Source: CAD feature listing. Evaluate the final solid. Frame: model axes, mm. A direction names the side the tool comes from. Coordinates: 2 decimals unless noted, no trailing zeros. Loops run counter-clockwise (first coordinate to the right, second up) from the corner with the lowest first, then second, coordinate; pieces in that order, holes last.
from build123d import *

# Parameters (mm, degrees)
BOSS_EXTRUDE1_DEPTH = 3.175
SKETCH2_R           = 2.5527
CUT_EXTRUDE1_DEPTH  = 77.793005053
SKETCH3_R           = 2.5527
CUT_EXTRUDE2_DEPTH  = 77.793005053


with BuildPart() as part:
    # Sketch1 → Boss-Extrude1 (new body)
    with BuildSketch(Plane(origin=(0, 0, 0), x_dir=(1, 0, 0), z_dir=(0, 1, 0))):
        Polygon((0, 0), (0, 44.45), (-13.97, 44.45), (-13.97, 67.31), (36.83, 67.31), (36.83, 44.45), (22.86, 44.45), (22.86, 0), align=None)
    extrude(amount=BOSS_EXTRUDE1_DEPTH)

    # Sketch2 → Cut-Extrude1 (cut, through all)
    with BuildSketch(Plane(origin=(0, 3.175, 0), x_dir=(1, 0, 0), z_dir=(0, 1, 0))):
        with Locations(Location((-7.62, 57.15, 0), (0, 0, 270))):
            Circle(SKETCH2_R)
        with Locations(Location((5.08, 57.15, 0), (0, 0, 270))):
            Circle(SKETCH2_R)
        with Locations(Location((17.78, 57.15, 0), (0, 0, 270))):
            Circle(SKETCH2_R)
        with Locations(Location((30.48, 57.15, 0), (0, 0, 270))):
            Circle(SKETCH2_R)
    extrude(amount=-CUT_EXTRUDE1_DEPTH, mode=Mode.SUBTRACT)

    # Sketch3 → Cut-Extrude2 (cut, through all)
    with BuildSketch(Plane(origin=(0, 3.175, 0), x_dir=(1, 0, 0), z_dir=(0, 1, 0))):
        with Locations(Location((11.43, 31.75, 0), (0, 0, 270))):
            Circle(SKETCH3_R)
        with Locations(Location((11.43, 19.05, 0), (0, 0, 270))):
            Circle(SKETCH3_R)
        with Locations(Location((11.43, 6.35, 0), (0, 0, 270))):
            Circle(SKETCH3_R)
    extrude(amount=-CUT_EXTRUDE2_DEPTH, mode=Mode.SUBTRACT)


solid = part.part
Q1. Section A-A, the plane x = 11.43. Return the cut outline in (y, z) (3 decimals).
Q2. Contact query for flat-ended pins moving along their axis: pin 1 Ø8 at (x, z) = (11.43, -19.05) entering from +Y (3 decimals); pin 2 Ø1.6 at (x, y) = (-7.5, 2.5) entering from +Z; pin 3 Ø1.6 at (y, z) = (2, -18) entering from -X. Output: stop coordinate, or through.
Q3. Section D-D, the plane x = 17.78. Return the cut outline in (y, z) (3 decimals), plus the area to 4 significant figures.
Q4. Draft query along X for faces 4 (the cylindrical face through (10.452, 1.61, -29.392)), 5 (the flat face through (0, 2, -22)), 6 (the flat face through (12, 3.175, -42)). Return one class per face: +X half, -X half, draft (parallel to the pull), parting line (faces both ways), or undercut.
Q5. Access query for faces 1 (the flat face through (12, 2, 0)), 2 (the flat face through (-7, 2, -44.45)), 3 (the flat face through (22.86, 2, -23)). Directions: +Z, -Z, +X, -X, +Y, -Y. A direction counts if a zero-diameter tool reaches every point of the face in a straight line with its end or side. Return the directions, or none.
Q6. Line query: line 1 along X through (y, z) = (1.6, -57.15); line 2 along X through (y, z) = (0.8, -19.05); line 3 along Z through (x, y) = (25.5, 2.5). Output: solid intervals per line, ascending.
Q7. Section B-B, the plane z = -6.35. Return the cut outline in (x, y) (3 decimals), plus the area to 3 significant figures.
Q8. Section C-C, the plane y = 2.15. Return the cut outline in (x, z).
Derived:
1. outline: (0, -67.31) - (3.175, -67.31) - (3.175, -34.303) - (0, -34.303) - close; (0, -29.197) - (3.175, -29.197) - (3.175, -21.603) - (0, -21.603) - close; (0, -16.497) - (3.175, -16.497) - (3.175, -8.903) - (0, -8.903) - close; (0, -3.797) - (3.175, -3.797) - (3.175, 0) - (0, 0) - close
2. pin 1: stops at y = 3.175
2. pin 2: stops at z = -44.45
2. pin 3: stops at x = 0
3. outline: (0, -67.31) - (3.175, -67.31) - (3.175, -59.703) - (0, -59.703) - close; (0, -54.597) - (3.175, -54.597) - (3.175, 0) - (0, 0) - close
3. area: 197.5 mm2
4. face 4: undercut
4. face 5: -X half
4. face 6: draft
5. face 1: +Z, +X, -X, +Y, -Y
5. face 2: +Z, -X, +Y, -Y
5. face 3: +Z, +X, +Y, -Y
6. line 1: x = -13.97 to -10.17, -5.07 to 2.53, 7.63 to 15.23, 20.33 to 27.93, 33.03 to 36.83
6. line 2: x = 0 to 8.88, 13.98 to 22.86
6. line 3: z = -67.31 to -44.45
7. outline: (0, 0) - (8.877, 0) - (8.877, 3.175) - (0, 3.175) - close; (13.983, 0) - (22.86, 0) - (22.86, 3.175) - (13.983, 3.175) - close
7. area: 56.4 mm2
8. outline: (-13.97, -67.31) - (36.83, -67.31) - (36.83, -44.45) - (22.86, -44.45) - (22.86, 0) - (0, 0) - (0, -44.45) - (-13.97, -44.45) - close; hole circle Ø5.11 at (-7.62, -57.15); hole circle Ø5.11 at (5.08, -57.15); hole circle Ø5.11 at (11.43, -31.75); hole circle Ø5.11 at (11.43, -19.05); hole circle Ø5.11 at (11.43, -6.35); hole circle Ø5.11 at (17.78, -57.15); hole circle Ø5.11 at (30.48, -57.15)
